Can you work these out from the model? Positions are in its coordinate system, mm. A direction names the side the tool comes from. Coordinates: 2 decimals unless noted, no trailing zeros. Order: outer loops, then holes, each group sorted by start corner. A loop starts at its lowest first (then second) coordinate and runs counter-clockwise, first axis right, second up. Notation, with made-up numbers: (3, 85.25) -> (60, 85.25) arc R19 cw to (60, 102.25) -> close; hole circle Ø1 at (53.25, 88.25). An arc over 180 degrees is marked (long way). Answer as a JSON object with one key per item and string values. Group by question number.
(1) I want a section at C-C, the plane x = 12.7. List the corners of the cut face in (y, z) for me (3 decimals), plus the area to 3 significant figures.
(2) I need wall thicknesses on line 1 (X direction, y = 12.25, z = 0) (3 decimals); line 2 (Y direction, x = 20.25, z = 0); line 3 (Y direction, x = 11, z = 0). Which ranges of each line are inside material? Lowest first, please.
(3) Which directions (+Z, -Z, +X, -X, +Y, -Y) give clear straight access to the entire face, cutting with the end or side of a thin tool? Please do faces 4 (the cylindrical face through (9.9, 12.4, 1.5)), 5 (the flat face through (25.4, 6, 3)).
(4) I want a section at D-D, the plane z = 4. List the corners of the cut face in (x, y) for me, plus the area to 3 significant figures.
(5) For pin 1 (4 mm diameter, centred on x = 5.5, z = -3, fed in from +Y); pin 2 (1.5 mm diameter, centred on y = 11, z = 0, fed in from -X) (3 decimals); pin 3 (5 mm diameter, centred on x = 18.5, y = -4, fed in from +Z), each with a flat end and sliding along its axis, tell me the tip position at first contact or that it passes through.
(6) I want a section at A-A, the plane z = 0. List the corners of the cut face in (x, y) for me (3 decimals), plus the area to 3 significant figures.
(7) I want a section at B-B, the plane y = 0. List the corners of the cut face in (x, z) for me.
(8) If we mould it in two halves opening along Y, with no side actions, what happens to faces 1 (the cylindrical face through (12.88, -6.2, 1.38)), 2 (the cylindrical face through (16.643, 12.53, -2.051)), 3 (the flat face through (16, 19.05, -2))? For each: pulls with the +Y half, pulls with the -Y half, needs draft (parallel to the pull), parting line crosses it, or undercut.
from build123d import *

# Parameters (mm, degrees)
SKETCH1_R               = 7.62
BOSS_EXTRUDE1_DEPTH     = 25.4
SKETCH2_R               = 4.445
BOSS_EXTRUDE2_DEPTH     = 19.05
SKETCH3_R               = 6.35
CUT_EXTRUDE1_DEPTH      = 33.651598895
CUT_EXTRUDE2_REACH      = 39.61
CUT_EXTRUDE2_END_RADIUS = 6.35
SKETCH4_R               = 3.175


with BuildPart() as part:
    # Sketch1 → Boss-Extrude1 (new body)
    with BuildSketch(Plane(origin=(0, 0, 0), x_dir=(0, 0, -1), z_dir=(1, 0, 0))):
        Circle(SKETCH1_R)
    extrude(amount=BOSS_EXTRUDE1_DEPTH)

    # Sketch2 → Boss-Extrude2 (add)
    with BuildSketch(Plane(origin=(0, 0, 0), x_dir=(1, 0, 0), z_dir=(0, 1, 0))):
        with Locations(Location((12.7, 0, 0), (0, 0, 90))):
            Circle(SKETCH2_R)
    extrude(amount=BOSS_EXTRUDE2_DEPTH)

    # Sketch3 → Cut-Extrude1 (cut, through all)
    with BuildSketch(Plane(origin=(25.4, 0, 0), x_dir=(0, 0, -1), z_dir=(1, 0, 0))):
        Circle(SKETCH3_R)
    extrude(amount=-CUT_EXTRUDE1_DEPTH, mode=Mode.SUBTRACT)

    # Cut-Extrude2: up to this cylinder (the profile starts outside it)
    cut_extrude2_end = Plane(origin=(12.7, 0, 0), z_dir=(1, 0, 0)) * Cylinder(CUT_EXTRUDE2_END_RADIUS, 92.92, mode=Mode.PRIVATE)
    # Sketch4 → Cut-Extrude2 (cut, up to the surface)
    with BuildSketch(Plane(origin=(0, 19.05, 0), x_dir=(1, 0, 0), z_dir=(0, 1, 0)), mode=Mode.PRIVATE) as cut_extrude2_sk1:
        with Locations(Location((12.7, 0, 0), (0, 0, 270))):
            Circle(SKETCH4_R)
    cut_extrude2_tool1 = extrude(cut_extrude2_sk1.sketch, amount=-CUT_EXTRUDE2_REACH, mode=Mode.PRIVATE) - cut_extrude2_end
    add(cut_extrude2_tool1.solids().sort_by_distance((12.7, 19.05, 0))[0], mode=Mode.SUBTRACT)


solid = part.part
Computed values:
{
 "1": {"outline": "(5.499, -3.175) arc R6.35 cw (long way) to (5.499, 3.175) -> (19.05, 3.175) -> (19.05, 4.445) -> (6.189, 4.445) arc R7.62 ccw (long way) to (6.189, -4.445) -> (19.05, -4.445) -> (19.05, -3.175) -> close", "area": "79.0 mm2"},
 "2": {"line 1": "x = 8.255 to 9.525, 15.875 to 17.145", "line 2": "y = -7.62 to -6.35, 6.35 to 7.62", "line 3": "y = -7.62 to -6.35"},
 "3": {"face 4": "+Y", "face 5": "+Z, -Z, +X, +Y, -Y"},
 "4": {"outline": "(0, -6.49) -> (25.4, -6.49) -> (25.4, -4.93) -> (0, -4.93) -> close; (0, 4.93) -> (25.4, 4.93) -> (25.4, 6.49) -> (14.64, 6.49) -> (14.64, 19.05) -> (10.76, 19.05) -> (10.76, 6.49) -> (0, 6.49) -> close", "area": "128 mm2"},
 "5": {"pin 1": "stops at y = 7.55", "pin 2": "stops at x = 8.255", "pin 3": "stops at z = 7.47"},
 "6": {"outline": "(0, -7.62) -> (25.4, -7.62) -> (25.4, -6.35) -> (0, -6.35) -> close; (0, 6.35) -> (9.525, 6.35) -> (9.525, 19.05) -> (8.255, 19.05) -> (8.255, 7.62) -> (0, 7.62) -> close; (15.875, 6.35) -> (25.4, 6.35) -> (25.4, 7.62) -> (17.145, 7.62) -> (17.145, 19.05) -> (15.875, 19.05) -> close", "area": "85.5 mm2"},
 "7": {"outline": "(0, -7.62) -> (25.4, -7.62) -> (25.4, -6.35) -> (0, -6.35) -> close; (0, 6.35) -> (25.4, 6.35) -> (25.4, 7.62) -> (0, 7.62) -> close"},
 "8": {"face 1": "undercut", "face 2": "needs draft", "face 3": "pulls with the +Y half"}
}
